from build123d import *

# Parameters (mm, degrees)
SKETCH_1_W               = 33
SKETCH_1_H               = 14
EXTRUDE_1_DEPTH          = 14
SKETCH_2_W               = 10
SKETCH_2_H               = 12
CUT_EXTRUDE_1_DEPTH      = 25.3
SKETCH_3_R               = 2
CUT_EXTRUDE_2_DEPTH      = 25.5
SKETCH_7_R               = 5
SKETCH_7_R_2             = 1.6
EXTRUDE_4_DEPTH          = 4
FILLET_4_DEPTH           = 14
SKETCH_8_R               = 4
SKETCH_8_R_2             = 1.6
EXTRUDE_5_DEPTH          = 7.3
SKETCH_10_R              = 2.5
EXTRUDE_6_DEPTH          = 4
CUT_EXTRUDE_3_DEPTH      = 26.401771619
CUT_EXTRUDE_3_DEPTH_BACK = 20


with BuildPart() as part:
    # 草图1 → 凸台-拉伸1 (new body)
    with BuildSketch(Plane(origin=(0, 0, 0), x_dir=(1, 0, 0), z_dir=(0, 1, 0))):
        Rectangle(SKETCH_1_W, SKETCH_1_H)
    extrude(amount=EXTRUDE_1_DEPTH)

    # 草图2 → 切除-拉伸1 (cut)
    with BuildSketch(Plane.ZY.offset(16.5)):
        with Locations((0, 7)):
            Rectangle(SKETCH_2_W, SKETCH_2_H)
    extrude(amount=-CUT_EXTRUDE_1_DEPTH, mode=Mode.SUBTRACT)

    # 草图3 → 切除-拉伸2 (cut)
    with BuildSketch(Plane(origin=(16.5, 0, 0), x_dir=(0, 0, -1), z_dir=(1, 0, 0))):
        with Locations((0, 10.5)):
            Circle(SKETCH_3_R)
        with Locations((0, 3.5)):
            Circle(SKETCH_3_R)
    extrude(amount=-CUT_EXTRUDE_2_DEPTH, mode=Mode.SUBTRACT)

    # 草图7 → 凸台-拉伸4 (add)
    with BuildSketch(Plane(origin=(0, 14, 0), x_dir=(1, 0, 0), z_dir=(0, 1, 0))):
        with Locations(Location((-8.5, 0, 0), (0, 0, 270))):
            Circle(SKETCH_7_R)
        with Locations(Location((-8.5, 0, 0), (0, 0, 270))):
            Circle(SKETCH_7_R_2, mode=Mode.SUBTRACT)
    extrude(amount=EXTRUDE_4_DEPTH)

    # 圆角4: read off the stored shape, not the designer's step
    # 圆角4 outline → 圆角4 (cut)
    with BuildSketch(Plane(origin=(0, 0, 0), x_dir=(1, 0, 0), z_dir=(0, 1, 0))):
        with BuildLine():
            ThreePointArc((3.5, 7), (10.245368782, 5.113055385), (15.032562595, 0))
            ThreePointArc((15.032562595, 0), (10.245368782, -5.113055385), (3.5, -7))
            Line((3.5, -7), (16.5, -7))
            Line((16.5, -7), (16.5, 7))
            Line((16.5, 7), (3.5, 7))
        make_face()
    extrude(amount=FILLET_4_DEPTH, mode=Mode.SUBTRACT)

    # 草图8 → 凸台-拉伸5 (add)
    with BuildSketch(Plane(origin=(0, 14, 0), x_dir=(1, 0, 0), z_dir=(0, 1, 0))):
        with Locations(Location((9.5, 0, 0), (0, 0, 270))):
            Circle(SKETCH_8_R)
        with Locations(Location((9.5, 0, 0), (0, 0, 270))):
            Circle(SKETCH_8_R_2, mode=Mode.SUBTRACT)
    extrude(amount=EXTRUDE_5_DEPTH)

    # 草图10 → 凸台-拉伸6 (add)
    with BuildSketch(Plane.XZ):
        with Locations(Location((-8.5, 0, 0), (0, 0, 270))):
            Circle(SKETCH_10_R)
    extrude(amount=EXTRUDE_6_DEPTH)

    # 草图11 → 切除-拉伸3 (cut, two sides: drawn at the far end of the back side and taken through both)
    with BuildSketch(Plane(origin=(0, 14, 0), x_dir=(1, 0, 0), z_dir=(0, 1, 0)).offset(-CUT_EXTRUDE_3_DEPTH_BACK)):
        with BuildLine():
            Line((13.662777944, 2.1066605), (13.644074044, 0))
            Line((13.644074044, 0), (15.032562595, 0))
            ThreePointArc((15.032562595, 0), (14.398690512, 1.086504435), (13.662777944, 2.1066605))
        make_face()
        with BuildLine():
            Line((15.032562595, 0), (13.644074044, 0))
            Line((13.644074044, 0), (13.644074044, -2.130053001))
            ThreePointArc((13.644074044, -2.130053001), (14.39051998, -1.099054484), (15.032562595, 0))
        make_face()
    extrude(amount=CUT_EXTRUDE_3_DEPTH + CUT_EXTRUDE_3_DEPTH_BACK, mode=Mode.SUBTRACT)


solid = part.part
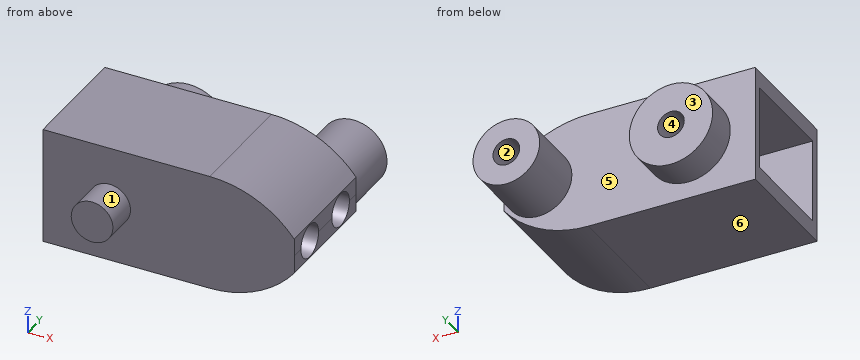
Build history of the part. All positions in model axes, mm. Face numbers are marked on the shaded views. A direction names the side the tool comes from. Round coordinates to 2 decimals unless told otherwise and drop trailing zeros. Write each loop counter-clockwise with the first axis right and the second up, starting at its lowest first coordinate (ties: lowest second). Pieces come first, ordered by that corner, then holes. Notation, with made-up numbers: M 27,68.25 L 53,68.25 A24 ccw 53,97.25 Z; hole C -14,20 d7. An arc over 180 degrees is marked long. Answer in a Markdown table with one row per item.
1. Saw through at B-B (y = 15.75). List the corners of the cut face in (x, z).
Geometry check:
| item | result |
|---|---|
| outline | C -8.5,0 d10; C 9.5,0 d8; hole C -8.5,0 d3.2; hole C 9.5,0 d3.2 |
2. Flat gauge pins, fed straight in: P1, Ø3, axis at x = -4, z = -5.5, coming from the +Y side; P2, Ø3, axis at x = -7, z = -2, coming from the +Y side; P3, Ø1.1, axis at y = 8, z = 1, coming from the +X side. Where does each tip first touch, or does it go through?
Geometry check:
| item | result |
|---|---|
| P1 | y = 14 |
| P2 | y = 18 |
| P3 | x = 13.64 |
3. Probe L1, parallel to X at y = 15.4, z = 0; L2, parallel to Y at x = -1, z = 0.75; L3, parallel to Z at x = -9, y = 10. List the from-to ranges inside material, lowest first. Write a range as [from, to].
Geometry check:
| item | result |
|---|---|
| L1 | [-13.5, -10.1], [-6.9, -3.5], [5.5, 7.9], [11.1, 13.5] |
| L2 | [0, 1], [13, 14] |
| L3 | [-7, -5], [5, 7] |
4. Mould opens along Z. For the marked faces 4, 5 and 6 say: +Z half, -Z half, draft (parallel to the pull), parting line (faces both ways), or undercut.
Geometry check:
| item | result |
|---|---|
| face 4 | undercut |
| face 5 | draft |
| face 6 | -Z half |
5. Saw through at A-A (x = -8.5). List the corners of the cut face in (y, z), and give its area (3 significant figures).
Geometry check:
| item | result |
|---|---|
| outline | M -4,-2.5 L 0,-2.5 L 0,-7 L 14,-7 L 14,-5 L 18,-5 L 18,-1.6 L 14,-1.6 L 14,1.6 L 18,1.6 L 18,5 L 14,5 L 14,7 L 0,7 L 0,2.5 L -4,2.5 Z; hole M 1,-5 L 13,-5 L 13,5 L 1,5 Z |
| area | 123 mm2 |
6. Saw through at D-D (z = 3). List the corners of the cut face in (x, y).
Geometry check:
| item | result |
|---|---|
| outline | M -16.5,0 L 12.88,0 L 12.88,14 L 12.15,14 L 12.15,21.3 L 6.85,21.3 L 6.85,14 L -4.5,14 L -4.5,18 L -12.5,18 L -12.5,14 L -16.5,14 L -16.5,13 L 8.8,13 L 8.8,1 L -16.5,1 Z |
7. Saw through at C-C (y = 3). List the corners of the cut face in (x, z), and give its area (3 significant figures).
Geometry check:
| item | result |
|---|---|
| outline | M -16.5,-7 L 3.5,-7 A13 ccw 13.66,-2.11 L 13.66,-1.94 L 8.8,-1.94 L 8.8,-5 L -16.5,-5 Z; M -16.5,5 L 8.8,5 L 8.8,1.94 L 13.64,1.94 L 13.64,2.13 A13 ccw 3.5,7 L -16.5,7 Z |
| area | 120 mm2 |
8. Which spindle directions (+Z, -Z, +X, -X, +Y, -Y) get a long thin tool onto all of the face, cutting with end or side? Do the marked faces 1, 2 and 3. Say none if no direction does.
Geometry check:
| item | result |
|---|---|
| face 1 | -Y |
| face 2 | +Y |
| face 3 | +Z, -Z, -X, +Y |
